The listing builds one solid part. Answer for the finished solid, in the listing's coordinates (mm). Give positions to 0.01 mm unless a question says otherwise; leave off trailing zeros. Write each loop counter-clockwise with the first axis right and the second up, starting at its lowest first coordinate (ties: lowest second). Pieces come first, ordered by that corner, then holes. Notation, with made-up numbers: (31, 41) - (60, 41) arc R16 cw to (60, 56) - close; hole circle Ø8 at (-30.5, 74.5). An arc over 180 degrees is marked (long way). Use a Markdown table: item, result. Add a question column.
from build123d import *

# Parameters (mm, degrees)
PAD_DEPTH = 270


with BuildPart() as part:
    # Sketch → Pad (new body)
    with BuildSketch(Plane.XY.offset(-458)):
        Polygon((212.856822, 82.967677), (213.717545, 84.06579), (217.886719, 80.797905), (219.106384, 82.400215), (214.944962, 85.586205), (215.26384, 85.984787), (218.771362, 86.431206), (222.094493, 83.872208), (221.12439, 78.232742), (225.725278, 76.87084), (226.231842, 80.657478), (230.660202, 77.31823), (231.115021, 73.836044), (230.812088, 73.413544), (226.654388, 76.597336), (225.42131, 75.008892), (229.506458, 71.832669), (228.64251, 70.721488), (223.935706, 70.128285), (213.440788, 78.259719), align=None)
    extrude(amount=PAD_DEPTH)


solid = part.part
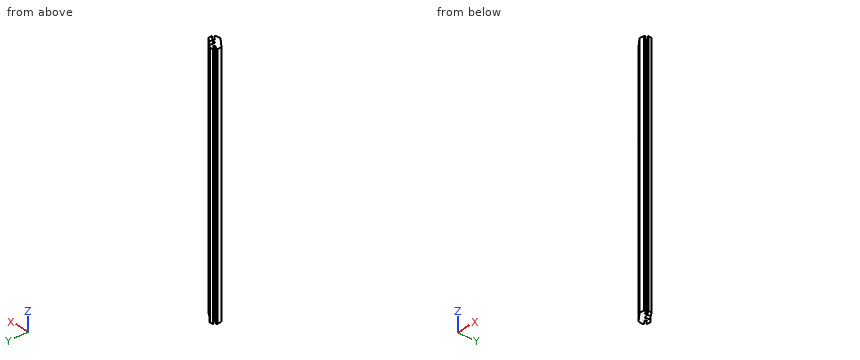
1. Consider L1, parallel to X at y = 79, z = -289; L2, parallel to Y at x = 218.75, z = -396.5; L3, parallel to X at y = 79.75, z = -397.5. Determine where each line is inside the solid, lowest interval first. Write a range as [from, to].
2. Given P1, Ø4, axis at y = 82.5, z = -244.5, coming from the +X side; P2, Ø2, axis at y = 78.5, z = -251.5, coming from the -X side; P3, Ø1.5, axis at y = 74.5, z = -286.5, coming from the -X side, each flat-ended and moving along its own axis, determine where each tip first touches the part or whether it passes through.
3. The part is cut by section A-A (z = -319). Give the vertices of the cut face in (x, y), and give its area (3 significant figures).
Check values:
| question | item | result |
|---|---|---|
| 1 | L1 | x = [213.35, 221.26], [226.01, 228.43] |
| 1 | L2 | y = [74.15, 81.93], [82.67, 86.43] |
| 1 | L3 | x = [213.26, 221.39], [226.11, 227.44] |
| 2 | P1 | stops at x = 226.44 |
| 2 | P2 | stops at x = 213.29 |
| 2 | P3 | stops at x = 217.33 |
| 3 | outline | (212.86, 82.97) - (213.44, 78.26) - (223.94, 70.13) - (228.64, 70.72) - (229.51, 71.83) - (225.42, 75.01) - (226.65, 76.6) - (230.81, 73.41) - (231.12, 73.84) - (230.66, 77.32) - (226.23, 80.66) - (225.73, 76.87) - (221.12, 78.23) - (222.09, 83.87) - (218.77, 86.43) - (215.26, 85.98) - (214.94, 85.59) - (219.11, 82.4) - (217.89, 80.8) - (213.72, 84.07) - close |
| 3 | area | 134 mm2 |
